Can you work these out from the drawing? Everything is in mm from the part's minimum corner. Give positions to 0.01 mm unless a question says otherwise; leave off trailing zeros. Order: outer loops, then holes, each group sorted by start corner. A loop starts at its lowest first (then second) coordinate and runs counter-clockwise, first axis right, second up. Notation, with made-up numbers: (0, 78) - (55, 78) arc R9 cw to (55, 86) - close; hole circle Ø11 at (31.25, 72.25). An arc over 180 degrees is marked (long way). One line per question, with ' | ' between items.
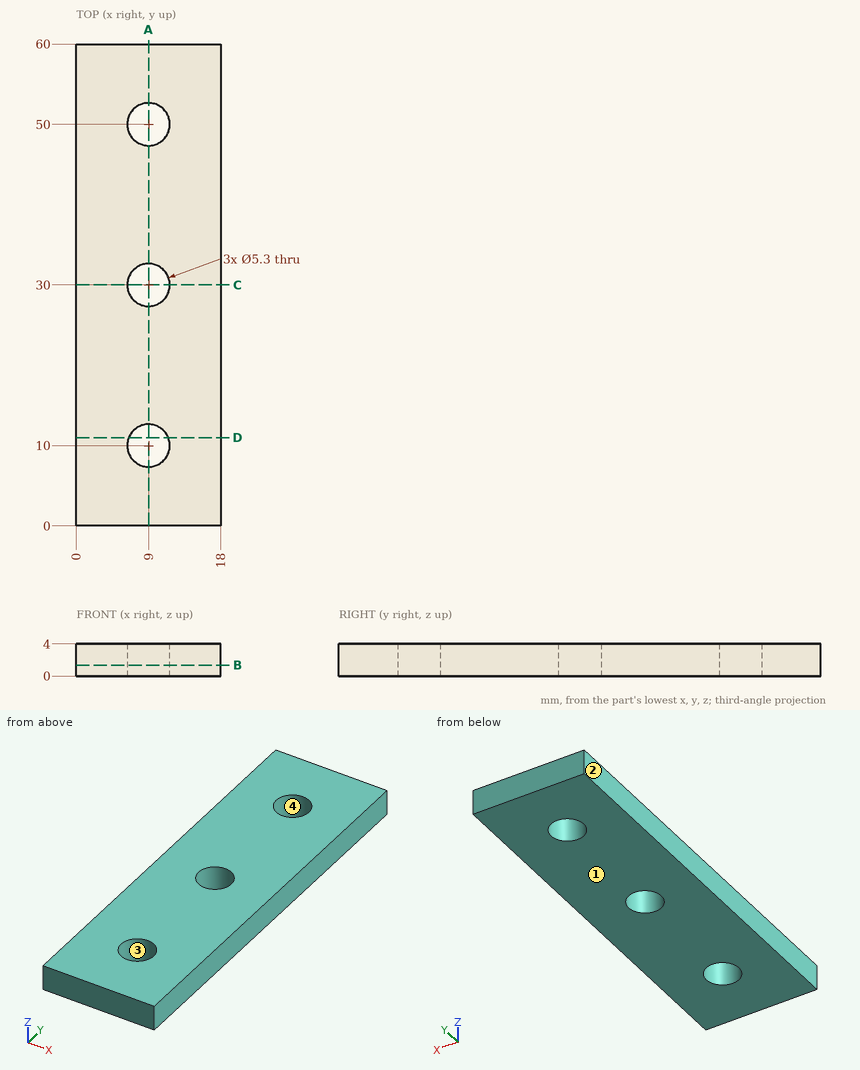
(1) If we mould it in two halves opening along X, with no side actions, what happens to the marked faces 1, 2, 3 and 4? For each: released by +X, released by -X, zero draft, split by the parting line, or undercut.
Answer below:
face 1: zero draft | face 2: released by -X | face 3: undercut | face 4: undercut
(2) If I drill on line 1 (Y direction, x = 9, z = 1.2); line 2 (Y direction, x = 8, z = 1.95); line 3 (X direction, y = 51, z = 1.9), over which ranges is the centre line in solid material (lowest first)?
Answer below:
line 1: 0 to 7.35, 12.65 to 27.35, 32.65 to 47.35, 52.65 to 60 | line 2: 0 to 7.55, 12.45 to 27.55, 32.45 to 47.55, 52.45 to 60 | line 3: 0 to 6.55, 11.45 to 18
(3) Imagine slicing it at B-B (z = 1.35). List the corners of the cut face in (x, y) for me.
Answer below:
outline: (0, 0) - (18, 0) - (18, 60) - (0, 60) - close; hole circle Ø5.3 at (9, 10); hole circle Ø5.3 at (9, 30); hole circle Ø5.3 at (9, 50)
(4) Imagine slicing it at C-C (y = 30). List the corners of the cut face in (x, z) for me, and give its area (3 significant figures).
Answer below:
outline: (0, 0) - (6.35, 0) - (6.35, 4) - (0, 4) - close; (11.65, 0) - (18, 0) - (18, 4) - (11.65, 4) - close | area: 50.8 mm^2
(5) Will this pin go through, and if not, where does the flat tip stop? pin 1 (4 mm diameter, centred on x = 9, y = 50, fed in from -Z).
Answer below:
pin 1: through
(6) Imagine slicing it at A-A (x = 9). List the corners of the cut face in (y, z) for me, and give its area (3 significant figures).
Answer below:
outline: (0, 0) - (7.35, 0) - (7.35, 4) - (0, 4) - close; (12.65, 0) - (27.35, 0) - (27.35, 4) - (12.65, 4) - close; (32.65, 0) - (47.35, 0) - (47.35, 4) - (32.65, 4) - close; (52.65, 0) - (60, 0) - (60, 4) - (52.65, 4) - close | area: 176 mm^2
(7) Imagine slicing it at D-D (y = 11). List the corners of the cut face in (x, z) for me, and give its area (3 significant figures).
Answer below:
outline: (0, 0) - (6.55, 0) - (6.55, 4) - (0, 4) - close; (11.45, 0) - (18, 0) - (18, 4) - (11.45, 4) - close | area: 52.4 mm^2
